Drawing for the job (mm, zero at the part's lowest x, y, z). Round coordinates to 2 decimals unless told otherwise and drop trailing zeros. Loops run counter-clockwise (first coordinate to the right, second up) from the corner with the lowest first, then second, coordinate; pieces in that order, holes last. Notation, with made-up numbers: (83, 7) -> (94, 7) arc R31 ccw to (94, 40) -> close; hole circle Ø6 at (55, 18). An arc over 180 degrees is marked (long way). Put each result on its own line as item: value. Start each with the question number.
Item 1: Pull direction X, two halves, no side cores. Call the marked faces 1, 2 and 3: +X half, -X half, draft (parallel to the pull), parting line (faces both ways), or undercut.
Item 2: Cut at A-A, the plane z = 2.4. List the corners of the cut face in (x, y) (1 decimal), plus the area to 3 significant figures.
Item 3: Cut at C-C, the plane x = 27.5. List the corners of the cut face in (y, z) (1 decimal).
Item 4: Flat gauge pin, fed straight in: pin 1 Ø1.5 at (y, z) = (19.5, 2) entering from -X. Where does the tip first touch, or does it go through?
Item 5: Cut at D-D, the plane y = 9. List the corners of the cut face in (x, z) (1 decimal).
Item 6: Drill centre lines: probe 1 along X at (y, z) = (22.5, 3); probe 2 along X at (y, z) = (13.5, 1.85) (1 decimal); probe 3 along X at (y, z) = (14, 2.45). Where is each one in solid material? Low to high. Write a range as [from, to].
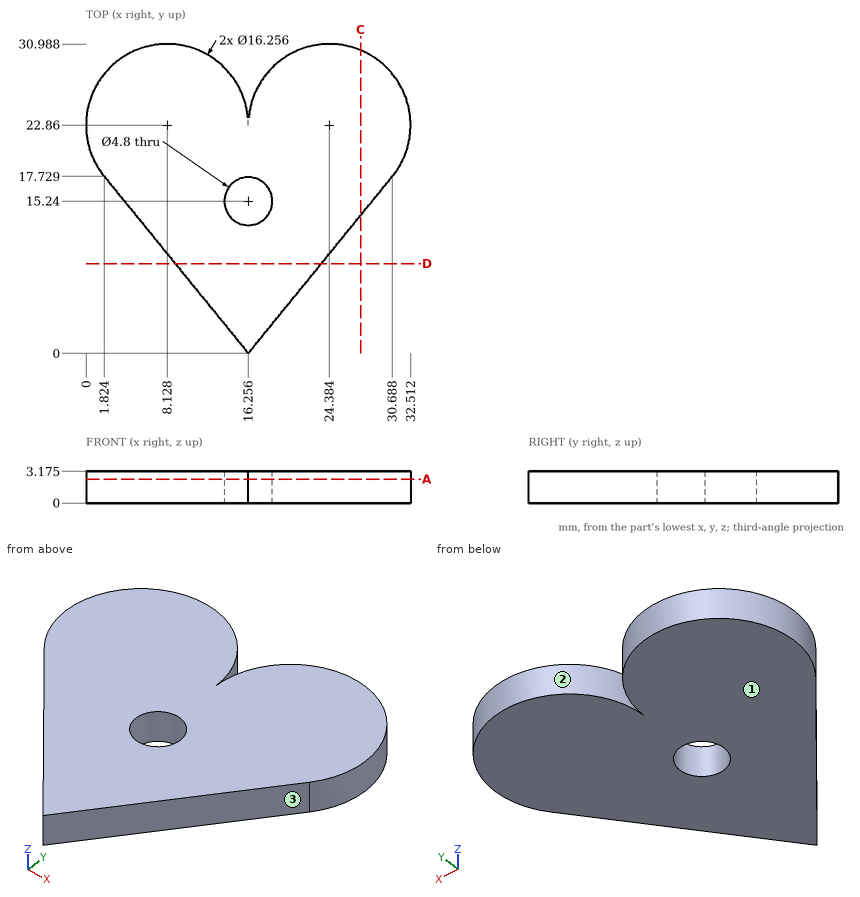
Reply:
1. face 1: draft
1. face 2: undercut
1. face 3: +X half
2. outline: (1.8, 17.7) -> (16.3, 0) -> (30.7, 17.7) arc R8.1 ccw (long way) to (16.3, 22.9) arc R8.1 ccw (long way) to start; hole circle Ø4.8 at (16.3, 15.2)
2. area: 606 mm^2
3. outline: (13.8, 0) -> (30.4, 0) -> (30.4, 3.2) -> (13.8, 3.2) -> close
4. pin 1: stops at x = 0.43
5. outline: (8.9, 0) -> (23.6, 0) -> (23.6, 3.2) -> (8.9, 3.2) -> close
6. probe 1: x = [0.01, 32.5]
6. probe 2: x = [5.3, 14.6], [17.9, 27.2]
6. probe 3: x = [4.86, 14.2], [18.31, 27.65]
